```python
from build123d import *

# Parameters (mm, degrees)
SKETCH_1_R                  = 2.5
EXTRUDE_1_DEPTH             = 2
SKETCH_2_R                  = 2
EXTRUDE_3_DEPTH             = 2
EXTRUDE_4_REACH             = 93.431
SKETCH_4_R                  = 4
EXTRUDE_5_REACH             = 93.431
EXTRUDE_6_REACH             = 56.956
EXTRUDE_6_DIRECTION_2_DEPTH = 3


with BuildPart() as part:
    # Sketch 1 → Extrude 1 (new body)
    with BuildSketch(Plane(origin=(0, 0, 0), x_dir=(1, 0, 0), z_dir=(0, 1, 0))):
        Polygon((10.502525317, -60), (60, -10.502525317), (60, 0), (20, 0), (20, -20), (0, -20), (0, -60), align=None)
        with Locations(Location((10, -52, 0), (0, 0, 270))):
            Circle(SKETCH_1_R, mode=Mode.SUBTRACT)
        with Locations(Location((52, -10, 0), (0, 0, 270))):
            Circle(SKETCH_1_R, mode=Mode.SUBTRACT)
    extrude(amount=EXTRUDE_1_DEPTH)



with BuildPart() as body_2:
    # Sketch 2 → Extrude 3 (new body)
    with BuildSketch(Plane(origin=(24.318415307, 24.081140456, 24.318415307), x_dir=(-0.7071067811865475, 0, 0.7071067811865476), z_dir=(0.5792279653395701, 0.5735764363510444, 0.57922796533957))):
        Polygon((-3, 16.786030205), (-15, 16.786030205), (-15, -13.213969795), (15, -13.213969795), (15, 9.786030205), (-3, 9.786030205), align=None)
        with Locations(Location((-12, -10.213969795, 0), (0, 0, 180))):
            Circle(SKETCH_2_R, mode=Mode.SUBTRACT)
        with Locations(Location((12, -10.213969795, 0), (0, 0, 180))):
            Circle(SKETCH_2_R, mode=Mode.SUBTRACT)
        with Locations(Location((-12, 13.786030205, 0), (0, 0, 180))):
            Circle(SKETCH_2_R, mode=Mode.SUBTRACT)
    extrude(amount=EXTRUDE_3_DEPTH)


with BuildPart() as part_1:
    add(part.part)

    add(body_2.part)  # Extrude 4 merges body 2
    # Extrude 4: up to this plane
    extrude_4_end = Plane(origin=(24.318415307, 24.081140456, 24.318415307), z_dir=(0.5792279653395702, 0.5735764363510445, 0.5792279653395699))
    # Sketch 4 → Extrude 4 (add, up to the surface)
    with BuildSketch(Plane(origin=(0, 2, 0), x_dir=(1, 0, 0), z_dir=(0, 1, 0)), mode=Mode.PRIVATE) as extrude_4_sk1:
        with Locations(Location((26.030164055, -18.959096243, 0), (0, 0, 315))):
            Circle(SKETCH_4_R)
    extrude_4_tool1 = split(extrude(extrude_4_sk1.sketch, amount=EXTRUDE_4_REACH, mode=Mode.PRIVATE), bisect_by=extrude_4_end, keep=Keep.BOTH, mode=Mode.PRIVATE)
    add(extrude_4_tool1.solids().sort_by_distance((26.030164, 2, 18.959096))[0])

    # Sketch 5 → Extrude 5 (add, up to next)
    with BuildSketch(Plane(origin=(0, 2, 0), x_dir=(1, 0, 0), z_dir=(0, 1, 0)), mode=Mode.PRIVATE) as extrude_5_sk1:
        Polygon((41.733091591, -20.519888156), (33.247810217, -29.00516953), (34.406266148, -30.16362546), (42.891547522, -21.678344086), align=None)
    extrude_5_tool1 = extrude(extrude_5_sk1.sketch, amount=EXTRUDE_5_REACH, mode=Mode.PRIVATE) - part_1.part
    add(extrude_5_tool1.solids().sort_by_distance((38.069679, 2, 25.341757))[0])

    # Extrude 6: up to this face of the body (flat: up to its plane)
    extrude_6_end = Plane(part_1.part.faces().sort_by_distance((24.757422588, 23.562214363, 24.393270957))[0])
    # Sketch 6 → Extrude 6 (add, up to the picked face)
    with BuildSketch(Plane(origin=(25.476871238, 25.228293329, 25.476871238), x_dir=(0.45107473692648714, 0.36633593098762024, -0.8138363271408656), z_dir=(0.5792279653395701, 0.5735764363510444, 0.5792279653395701)), mode=Mode.PRIVATE) as extrude_6_sk1:
        Polygon((-7.506940922, 18.527137818), (-17.792853619, -2.044687575), (-19.581708001, -1.150260384), (-9.295795304, 19.421565009), align=None)
    extrude_6_tool1 = split(extrude(extrude_6_sk1.sketch, amount=-EXTRUDE_6_REACH, mode=Mode.PRIVATE), bisect_by=extrude_6_end, keep=Keep.BOTH, mode=Mode.PRIVATE)
    # Sketch 6 → Extrude 6 (add, up to the picked face)
    with BuildSketch(Plane(origin=(25.476871238, 25.228293329, 25.476871238), x_dir=(0.45107473692648714, 0.36633593098762024, -0.8138363271408656), z_dir=(0.5792279653395701, 0.5735764363510444, 0.5792279653395701)), mode=Mode.PRIVATE) as extrude_6_sk2:
        Polygon((19.325874808, 5.110729953), (5.909466943, -21.722085777), (7.698321325, -22.616512968), (21.11472919, 4.216302762), align=None)
    extrude_6_tool2 = split(extrude(extrude_6_sk2.sketch, amount=-EXTRUDE_6_REACH, mode=Mode.PRIVATE), bisect_by=extrude_6_end, keep=Keep.BOTH, mode=Mode.PRIVATE)
    add(extrude_6_tool1.solids().sort_by(Axis((13.468011, 26.632295, 36.095428), (-0.5792279653395701, -0.5735764363510444, -0.5792279653395701)))[0])
    add(extrude_6_tool2.solids().sort_by(Axis((37.514957, 23.765263, 14.88754), (-0.5792279653395701, -0.5735764363510444, -0.5792279653395701)))[0])

    # Sketch 6 → Extrude 6 direction 2 (add)
    with BuildSketch(Plane(origin=(25.476871238, 25.228293329, 25.476871238), x_dir=(0.45107473692648714, 0.36633593098762024, -0.8138363271408656), z_dir=(0.5792279653395701, 0.5735764363510444, 0.5792279653395701))):
        Polygon((-7.506940922, 18.527137818), (-17.792853619, -2.044687575), (-19.581708001, -1.150260384), (-9.295795304, 19.421565009), align=None)
        Polygon((19.325874808, 5.110729953), (5.909466943, -21.722085777), (7.698321325, -22.616512968), (21.11472919, 4.216302762), align=None)
    extrude(amount=EXTRUDE_6_DIRECTION_2_DEPTH)


solid = part_1.part
```
Verification items for the finished model (mm, model axes). A direction names the side the tool comes from. Round coordinates to 2 decimals unless told otherwise and drop trailing zeros. Write each loop counter-clockwise with the first axis right and the second up, starting at its lowest first coordinate (ties: lowest second). Pieces come first, ordered by that corner, then holes. Notation, with made-up numbers: (17, 38.25) - (75, 38.25) arc R17 ccw to (75, 44.25) - close; hole circle Ø5 at (-28.5, 38). An arc over 180 degrees is marked (long way). Answer as a JSON object with one key per item and string values. Group by question number.
Q1. Go/stop test with flat-tipped pins: pin 1 Ø18 at (x, z) = (15.5, 20.5) entering from +Y; pin 2 Ø8 at (x, z) = (52, 6.5) entering from -Y; pin 3 Ø6 at (x, y) = (22.5, 29.5) entering from -Z; pin 4 Ø2 at (x, z) = (45, 11.5) entering from +Y. Record where each tip stops, or that it passes through.
Q2. Section check A-A, the plane x = 52. Enter the section's corners in (y, z).
Q3. Section check C-C, the plane z = 52. Enter the section's corners in (x, y), plus the area to 3 significant figures.
Q4. Mould release check, pull along Y, two halves, no side actions. Record for faces 1 (the flat face through (10, 1, 20)), 2 (the flat face through (39.193, 25.52, 16.651)), 3 (the cylindrical face through (23.33, 14.11, 16.01)): released by +Y, released by -Y, zero draft, split by the parting line, or undercut.
Q5. Thickness scan on line 1 (X direction, y = 1.55, z = 10); line 2 (Y direction, x = 43.5, z = 25); line 3 (X direction, y = 1, z = 52). Record the ranges inside material, lowest first.
Q6. Tool access check on faces 4 (the flat face through (37.55, 6.107, 24.703)), 5 (the flat face through (37.579, 24.786, 16.366)), 6 (the flat face through (43.858, 11.745, 21.25)), 7 (the flat face through (38.62, 23.9, 14.58)). Record the directions out of +Z, -Z, +X, -X, +Y, -Y that give a thin tool (end or side, any length) a straight path to the whole face; none if there is none.
Q7. Section check D-D, the plane x = 35.5. Enter the section's corners in (y, z), plus the area to 3 significant figures.
Q8. Section check B-B, the plane y = 4. Enter the section's corners in (x, z), plus the area to 3 significant figures.
Found:
{
 "1": {"pin 1": "stops at y = 36.05", "pin 2": "stops at y = 0", "pin 3": "stops at z = 14.99", "pin 4": "stops at y = 2"},
 "2": {"outline": "(0, 0) - (2, 0) - (2, 7.5) - (0, 7.5) - close; (0, 12.5) - (2, 12.5) - (2, 18.5) - (0, 18.5) - close"},
 "3": {"outline": "(0, 0) - (7.5, 0) - (7.5, 2) - (0, 2) - close; (12.5, 0) - (18.5, 0) - (18.5, 2) - (12.5, 2) - close", "area": "27.0 mm^2"},
 "4": {"face 1": "zero draft", "face 2": "released by +Y", "face 3": "undercut"},
 "5": {"line 1": "x = 20 to 49.5, 54.5 to 60", "line 2": "y = 0 to 2", "line 3": "x = 0 to 7.5, 12.5 to 18.5"},
 "6": {"face 4": "-Z", "face 5": "+Z, +Y", "face 6": "+X", "face 7": "-Z, +X, +Y"},
 "7": {"outline": "(0, 0) - (2, 0) - (2, 26.75) - (10.33, 26.75) - (25.78, 11.46) - (34.49, 11.46) - (31.64, 14.29) - (26.41, 14.29) - (11.48, 29.07) - (2, 29.07) - (2, 35) - (0, 35) - close", "area": "163 mm^2"},
 "8": {"outline": "circle Ø8 at (26.03, 18.96); (33.25, 29.01) - (41.73, 20.52) - (42.89, 21.68) - (34.41, 30.16) - close", "area": "69.9 mm^2"}
}
